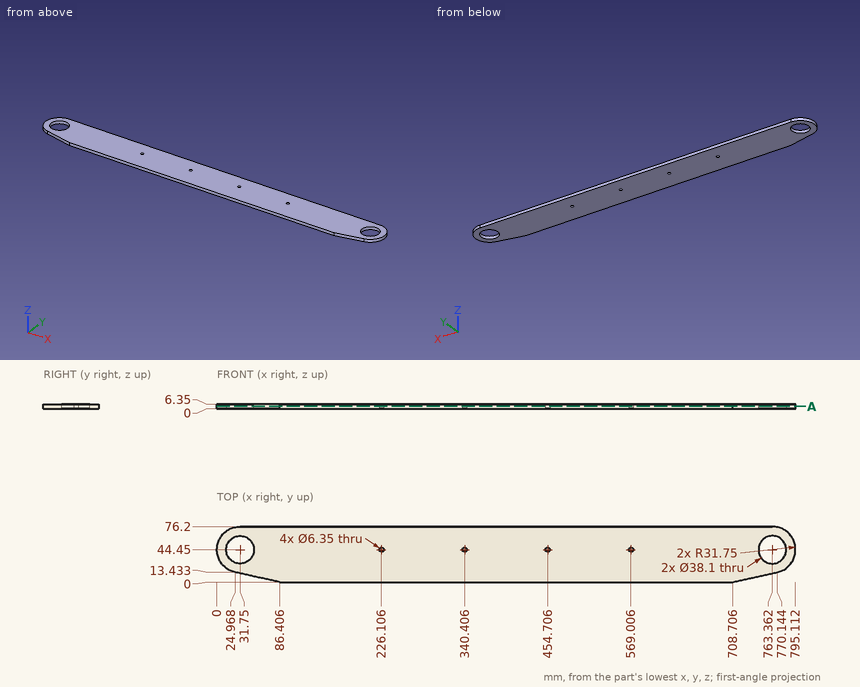
For this review, use the dimensioned drawing (mm, ordinates from the lowest corner) and the shaded views. Give positions to 0.01 mm unless a question says otherwise; leave off trailing zeros.
(1) To check wall thickness, follow L1, parallel to Y at x = 758, z = 1.25; L2, parallel to Y at x = 339, z = 2 (1 decimal); L3, parallel to X at y = 23, z = 1. State the ranges of each line that lie inside material, in increasing order.
(2) Consider section A-A, the plane z = 3.25. Give the number of separate pieces and of enclosed holes in the cut face, and give its area (3 significant figures).
(3) For P1, Ø4, axis at x = 569.01, y = 44.45, coming from the -Z side; P2, Ø3, axis at y = 51, z = 1, coming from the -X side, all flat-tipped, find the tip position at first contact; note any pin that passes through.
Returned:
1. L1: y = 10.78 to 26.17, 62.73 to 76.2
1. L2: y = 0 to 41.6, 47.3 to 76.2
1. L3: x = 8.34 to 786.77
2. separate pieces: 1
2. enclosed holes: 6
2. area: 55,900 mm2
3. P1: passes through
3. P2: stops at x = 0.4
